```python
from build123d import *

# Parameters (mm, degrees)
MODEL_R             = 3.6
MODEL_R_2           = 2.5
BOSS_EXTRUDE1_DEPTH = 3


with BuildPart() as part:
    # Model → Boss-Extrude1 (new body)
    with BuildSketch(Plane.XY):
        with BuildLine():
            Line((-63.589037408, 104.045286478), (-64.491971364, 103.346418738))
            Line((-64.491971364, 103.346418738), (-65.195294282, 102.464131076))
            Line((-65.195294282, 102.464131076), (-65.706925279, 101.376095796))
            Line((-65.706925279, 101.376095796), (-66.01810151, 100.051055017))
            Line((-66.01810151, 100.051055017), (-69.517848709, 75.149059762))
            Line((-69.517848709, 75.149059762), (-69.565467008, 73.768185024))
            Line((-69.565467008, 73.768185024), (-69.321374593, 72.25214776))
            Line((-69.321374593, 72.25214776), (-68.771556944, 70.621505836))
            Line((-68.771556944, 70.621505836), (-67.922379623, 68.902975774))
            Line((-67.922379623, 68.902975774), (-66.786009136, 67.108706641))
            Line((-66.786009136, 67.108706641), (-58.427898105, 55.121080623))
            ThreePointArc((-58.427898105, 55.121080623), (-58.113658938, 54.481447327), (-58.0056, 53.777032482))
            Line((-58.0056, 53.777032482), (-58.0056, 29.705859287))
            ThreePointArc((-58.0056, 29.705859287), (-58.113493434, 29.001971409), (-58.427266507, 28.362717471))
            Line((-58.427266507, 28.362717471), (-67.733176699, 15.002327604))
            Line((-67.733176699, 15.002327604), (-68.737483208, 13.38044762))
            Line((-68.737483208, 13.38044762), (-69.450197862, 11.816899792))
            Line((-69.450197862, 11.816899792), (-69.867580727, 10.329866757))
            Line((-69.867580727, 10.329866757), (-70, 8.951275064))
            Line((-70, 8.951275064), (-70, -8.799924936))
            ThreePointArc((-70, -8.799924936), (-69.01608381, -11.175308746), (-66.6407, -12.159224936))
            Line((-66.6407, -12.159224936), (-20.346130051, -12.159224936))
            ThreePointArc((-20.346130051, -12.159224936), (-19.542382714, -12.017502594), (-18.835579168, -11.609429377))
            Line((-18.835579168, -11.609429377), (-5.655220832, -0.549795559))
            ThreePointArc((-5.655220832, -0.549795559), (-4.948417286, -0.141722341), (-4.144669949, 0))
            Line((-4.144669949, 0), (4.144669949, 0))
            ThreePointArc((4.144669949, 0), (4.948417286, -0.141722341), (5.655220832, -0.549795559))
            Line((5.655220832, -0.549795559), (18.835579168, -11.609429377))
            ThreePointArc((18.835579168, -11.609429377), (19.542382714, -12.017502594), (20.346130051, -12.159224936))
            Line((20.346130051, -12.159224936), (66.64, -12.159224936))
            ThreePointArc((66.64, -12.159224936), (69.015878785, -11.17510372), (70, -8.799224936))
            Line((70, -8.799224936), (70, 8.951275064))
            Line((70, 8.951275064), (69.867655237, 10.329854089))
            Line((69.867655237, 10.329854089), (69.450510447, 11.816864236))
            Line((69.450510447, 11.816864236), (68.738189425, 13.380413155))
            Line((68.738189425, 13.380413155), (67.734411359, 15.002327604))
            Line((67.734411359, 15.002327604), (58.431323409, 28.365944307))
            ThreePointArc((58.431323409, 28.365944307), (58.117803534, 29.004991954), (58.01, 29.708593408))
            Line((58.01, 29.708593408), (58.01, 53.780426534))
            ThreePointArc((58.01, 53.780426534), (58.11796888, 54.484554688), (58.431954432, 55.123981627))
            Line((58.431954432, 55.123981627), (66.78348855, 67.108706641))
            Line((66.78348855, 67.108706641), (67.921135722, 68.90552929))
            Line((67.921135722, 68.90552929), (68.770985107, 70.624910502))
            Line((68.770985107, 70.624910502), (69.321132211, 72.254429785))
            Line((69.321132211, 72.254429785), (69.565833124, 73.768624559))
            Line((69.565833124, 73.768624559), (69.518710346, 75.149059762))
            Line((69.518710346, 75.149059762), (66.018963147, 100.051055017))
            Line((66.018963147, 100.051055017), (65.69880853, 101.401637743))
            Line((65.69880853, 101.401637743), (65.172247364, 102.501733058))
            Line((65.172247364, 102.501733058), (64.474805148, 103.363406486))
            Line((64.474805148, 103.363406486), (63.589037408, 104.045286478))
            Line((63.589037408, 104.045286478), (45.129929366, 115.221048558))
            ThreePointArc((45.129929366, 115.221048558), (44.544648343, 115.474250568), (43.912842483, 115.560775065))
            Line((43.912842483, 115.560775065), (20.346130051, 115.560775065))
            ThreePointArc((20.346130051, 115.560775065), (19.542382714, 115.419052723), (18.835579168, 115.010979506))
            Line((18.835579168, 115.010979506), (5.655220832, 103.951345688))
            ThreePointArc((5.655220832, 103.951345688), (4.948417286, 103.54327247), (4.144669949, 103.401550129))
            Line((4.144669949, 103.401550129), (-4.144669949, 103.401550129))
            ThreePointArc((-4.144669949, 103.401550129), (-4.948417286, 103.54327247), (-5.655220832, 103.951345688))
            Line((-5.655220832, 103.951345688), (-18.835579168, 115.010979506))
            ThreePointArc((-18.835579168, 115.010979506), (-19.542382714, 115.419052723), (-20.346130051, 115.560775065))
            Line((-20.346130051, 115.560775065), (-43.912842483, 115.560775065))
            ThreePointArc((-43.912842483, 115.560775065), (-44.544648343, 115.474250568), (-45.129929366, 115.221048558))
            Line((-45.129929366, 115.221048558), (-63.589037408, 104.045286478))
        make_face()
        with Locations((-56.5, 1.360775064)):
            Circle(MODEL_R, mode=Mode.SUBTRACT)
        with Locations((-10, 41.740775065)):
            Circle(MODEL_R_2, mode=Mode.SUBTRACT)
        with Locations((-39.85, 0.522775064)):
            Circle(MODEL_R_2, mode=Mode.SUBTRACT)
        with Locations((-39.85, 10.522775064)):
            Circle(MODEL_R_2, mode=Mode.SUBTRACT)
        with Locations((-39.85, 30.842775065)):
            Circle(MODEL_R_2, mode=Mode.SUBTRACT)
        with Locations((-39.85, 51.162775065)):
            Circle(MODEL_R_2, mode=Mode.SUBTRACT)
        with Locations((-31.925, 81.060775064)):
            Circle(MODEL_R_2, mode=Mode.SUBTRACT)
        with Locations((-39.85, 61.162775065)):
            Circle(MODEL_R_2, mode=Mode.SUBTRACT)
        with Locations((-39.85, 101.162775064)):
            Circle(MODEL_R_2, mode=Mode.SUBTRACT)
        with Locations((-56.5, 81.060775064)):
            Circle(MODEL_R_2, mode=Mode.SUBTRACT)
        with Locations((39.85, 0.522775064)):
            Circle(MODEL_R, mode=Mode.SUBTRACT)
        with Locations((39.85, 30.842775065)):
            Circle(MODEL_R, mode=Mode.SUBTRACT)
        with Locations((56.5, 1.360775064)):
            Circle(MODEL_R, mode=Mode.SUBTRACT)
        with Locations((10, 41.740775065)):
            Circle(MODEL_R_2, mode=Mode.SUBTRACT)
        with Locations((39.85, 10.522775064)):
            Circle(MODEL_R_2, mode=Mode.SUBTRACT)
        with Locations((39.85, 51.162775065)):
            Circle(MODEL_R_2, mode=Mode.SUBTRACT)
        with Locations((39.85, 61.162775065)):
            Circle(MODEL_R, mode=Mode.SUBTRACT)
        with Locations((39.85, 101.162775064)):
            Circle(MODEL_R, mode=Mode.SUBTRACT)
        with Locations((31.925, 81.060775064)):
            Circle(MODEL_R_2, mode=Mode.SUBTRACT)
        with Locations((56.5, 81.060775064)):
            Circle(MODEL_R_2, mode=Mode.SUBTRACT)
        with BuildLine():
            Line((-26.57, 98.240775065), (-26.57, 89.240775065))
            ThreePointArc((-26.57, 89.240775065), (-23.57, 86.240775065), (-20.57, 89.240775065))
            Line((-20.57, 89.240775065), (-20.57, 98.240775065))
            ThreePointArc((-20.57, 98.240775065), (-23.57, 101.240775065), (-26.57, 98.240775065))
        make_face(mode=Mode.SUBTRACT)
        with BuildLine():
            Line((-17.5, 72.80015), (-17.5, 66.89985))
            ThreePointArc((-17.5, 66.89985), (-14.849360304, 60.500639696), (-8.45015, 57.85))
            Line((-8.45015, 57.85), (8.45015, 57.85))
            ThreePointArc((8.45015, 57.85), (14.849360304, 60.500639696), (17.5, 66.89985))
            Line((17.5, 66.89985), (17.5, 72.80015))
            ThreePointArc((17.5, 72.80015), (14.849360304, 79.199360304), (8.45015, 81.85))
            Line((8.45015, 81.85), (-8.45015, 81.85))
            ThreePointArc((-8.45015, 81.85), (-14.849360304, 79.199360304), (-17.5, 72.80015))
        make_face(mode=Mode.SUBTRACT)
        with BuildLine():
            Line((20.57, 98.240775065), (20.57, 89.240775065))
            ThreePointArc((20.57, 89.240775065), (23.57, 86.240775065), (26.57, 89.240775065))
            Line((26.57, 89.240775065), (26.57, 98.240775065))
            ThreePointArc((26.57, 98.240775065), (23.57, 101.240775065), (20.57, 98.240775065))
        make_face(mode=Mode.SUBTRACT)
    extrude(amount=BOSS_EXTRUDE1_DEPTH)


solid = part.part
```
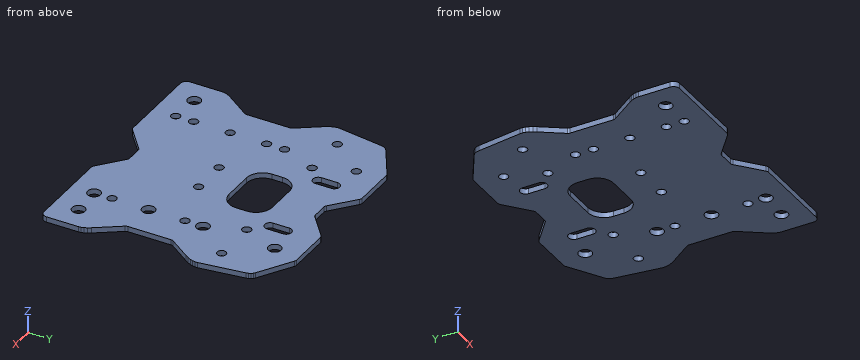
CAD build for the part. Positions are in the model's coordinates, mm. Coordinates: 2 decimals unless noted, no trailing zeros. Write each loop counter-clockwise with the first axis right and the second up, starting at its lowest first coordinate (ties: lowest second). Pieces come first, ordered by that corner, then holes.
(1) Drill centre lines: probe 1 along X at (y, z) = (94.5, 0.35); probe 2 along X at (y, z) = (50, 1.8); probe 3 along Y at (x, z) = (-57.5, 1.55). Where is each one in solid material? Low to high.
(2) Cut at C-C, the plane y = 91.5. List the corners of the cut face in (x, z).
(3) Cut at B-B, the plane x = 23.57. List the corners of the cut face in (y, z), and give its area (3 significant figures).
(4) Flat gauge pins, fed straight in: pin 1 (4.5 mm diameter, centred on x = -39.85, y = 101.16, fed in from -Z); pin 2 (1.5 mm diameter, centred on y = 70.5, z = 1.5, fed in from +X); pin 3 (0.9 mm diameter, centred on y = 94.5, z = 1.5, fed in from +X). Where does each tip first touch, or does it go through?
(5) Cut at A-A, the plane x = -39.85. List the corners of the cut face in (y, z), and give its area (3 significant figures).
(6) Cut at D-D, the plane x = 39.85. List the corners of the cut face in (y, z), and give its area (3 significant figures).
Geometry says:
1. probe 1: x = -66.8 to -26.57, -20.57 to 20.57, 26.57 to 66.8
1. probe 2: x = -58.01 to -42.06, -37.64 to 37.64, 42.06 to 58.01
1. probe 3: y = -12.16 to -2.1, 4.82 to 78.77, 83.35 to 107.73
2. outline: (-67.22, 0) - (-26.57, 0) - (-26.57, 3) - (-67.22, 3) - close; (-20.57, 0) - (20.57, 0) - (20.57, 3) - (-20.57, 3) - close; (26.57, 0) - (67.22, 0) - (67.22, 3) - (26.57, 3) - close
3. outline: (-12.16, 0) - (86.24, 0) - (86.24, 3) - (-12.16, 3) - close; (101.24, 0) - (115.56, 0) - (115.56, 3) - (101.24, 3) - close
3. area: 338 mm2
4. pin 1: passes through
4. pin 2: stops at x = 68.98
4. pin 3: stops at x = 66.86
5. outline: (-12.16, 0) - (-1.98, 0) - (-1.98, 3) - (-12.16, 3) - close; (3.02, 0) - (8.02, 0) - (8.02, 3) - (3.02, 3) - close; (13.02, 0) - (28.34, 0) - (28.34, 3) - (13.02, 3) - close; (33.34, 0) - (48.66, 0) - (48.66, 3) - (33.34, 3) - close; (53.66, 0) - (58.66, 0) - (58.66, 3) - (53.66, 3) - close; (63.66, 0) - (98.66, 0) - (98.66, 3) - (63.66, 3) - close; (103.66, 0) - (115.56, 0) - (115.56, 3) - (103.66, 3) - close
5. area: 293 mm2
6. outline: (-12.16, 0) - (-3.08, 0) - (-3.08, 3) - (-12.16, 3) - close; (4.12, 0) - (8.02, 0) - (8.02, 3) - (4.12, 3) - close; (13.02, 0) - (27.24, 0) - (27.24, 3) - (13.02, 3) - close; (34.44, 0) - (48.66, 0) - (48.66, 3) - (34.44, 3) - close; (53.66, 0) - (57.56, 0) - (57.56, 3) - (53.66, 3) - close; (64.76, 0) - (97.56, 0) - (97.56, 3) - (64.76, 3) - close; (104.76, 0) - (115.56, 0) - (115.56, 3) - (104.76, 3) - close
6. area: 267 mm2
